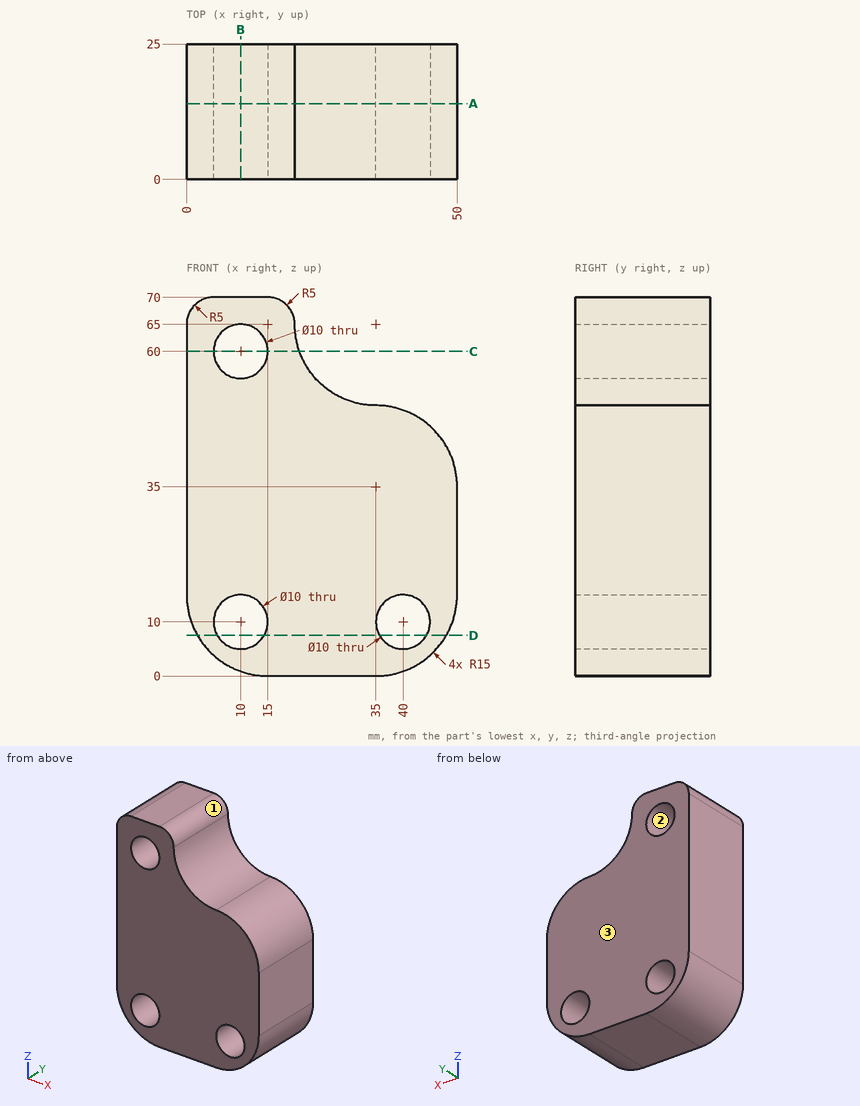
Here's the drawing with two shaded views (mm, measured from the low corner). I have some questions. Give positions to 0.01 mm unless a question says otherwise; leave off trailing zeros. Write each loop counter-clockwise with the first axis right and the second up, starting at its lowest first coordinate (ties: lowest second). Pieces come first, ordered by that corner, then holes. Notation, with made-up numbers: (62.5, 69) - (81.5, 69) arc R11 ccw to (81.5, 85) - close; hole circle Ø11 at (-5, -27.5). An arc over 180 degrees is marked (long way). One line per item, written item: value. Start each with the question number.
Item 1: Please list where these lines run through material, in increasing order: line 1 (Z direction, x = 13, y = 8.25); line 2 (Z direction, x = 10, y = 18.75); line 3 (X direction, y = 5.25, z = 5.5). Write a range as from..to.
Item 2: If we mould it in two halves opening along X, with no side actions, what happens to the marked faces 1, 2 and 3? For each: +X half, -X half, draft (parallel to the pull), parting line (faces both ways), or undercut.
Item 3: I'm going to push flat-ended pins straight in: pin 1 (4 mm diameter, centred on y = 2.5, z = 41, fed in from +X); pin 2 (11.5 mm diameter, centred on x = 40, z = 10, fed in from +Y); pin 3 (6 mm diameter, centred on x = 10, z = 10, fed in from +Y); pin 4 (1 mm diameter, centred on x = 43.5, y = 10, fed in from +Z). Where does each tip first touch, or does it pass through?
Item 4: Imagine slicing it at A-A, the plane y = 14. List the corners of the cut face in (x, z) for me.
Item 5: Imagine slicing it at B-B, the plane x = 10. List the corners of the cut face in (y, z) for me.
Item 6: Imagine slicing it at C-C, the plane z = 60. List the corners of the cut face in (x, y) for me.
Item 7: Imagine slicing it at D-D, the plane z = 7.5. List the corners of the cut face in (x, y) for me.
Geometry says:
1. line 1: 0.13..6, 14..56, 64..70
1. line 2: 0.86..5, 15..55, 65..70
1. line 3: 3.39..7.82, 12.18..37.82, 42.18..46.61
2. face 1: +X half
2. face 2: undercut
2. face 3: draft
3. pin 1: x = 49.46
3. pin 2: y = 25
3. pin 3: through
3. pin 4: z = 47.69
4. outline: (0, 15) arc R15 ccw to (15, 0) - (35, 0) arc R15 ccw to (50, 15) - (50, 35) arc R15 ccw to (35, 50) arc R15 cw to (20, 65) arc R5 ccw to (15, 70) - (5, 70) arc R5 ccw to (0, 65) - close; hole circle Ø10 at (10, 10); hole circle Ø10 at (10, 60); hole circle Ø10 at (40, 10)
5. outline: (0, 0.86) - (25, 0.86) - (25, 5) - (0, 5) - close; (0, 15) - (25, 15) - (25, 55) - (0, 55) - close; (0, 65) - (25, 65) - (25, 70) - (0, 70) - close
6. outline: (0, 0) - (5, 0) - (5, 25) - (0, 25) - close; (15, 0) - (20.86, 0) - (20.86, 25) - (15, 25) - close
7. outline: (2.01, 0) - (5.67, 0) - (5.67, 25) - (2.01, 25) - close; (14.33, 0) - (35.67, 0) - (35.67, 25) - (14.33, 25) - close; (44.33, 0) - (47.99, 0) - (47.99, 25) - (44.33, 25) - close
